Verification items for the finished model (mm, model axes). Face numbers are marked on the shaded views. A direction names the side the tool comes from. Round coordinates to 2 decimals unless told otherwise and drop trailing zeros. Order: outer loops, then holes, each group sorted by start corner. A loop starts at its lowest first (then second) coordinate and runs counter-clockwise, first axis right, second up.
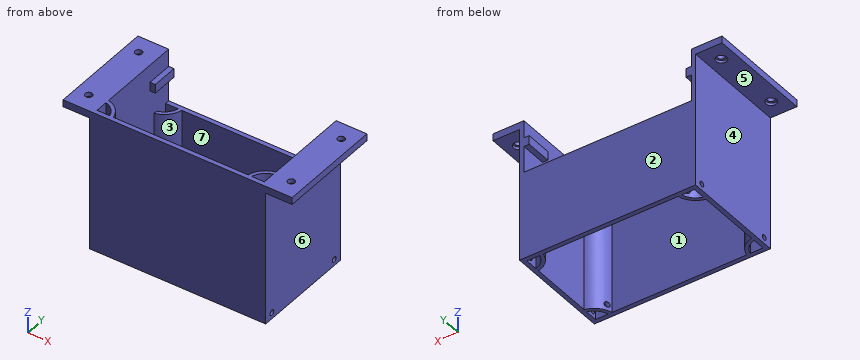
```python
from build123d import *

# Parameters (mm, degrees)
SKETCH1_W                = 100
SKETCH1_H                = 60
SKETCH1_W_2              = 95
SKETCH1_H_2              = 55
BOSS_EXTRUDE1_DEPTH      = 150
SKETCH2_W                = 95
SKETCH2_H                = 30
CUT_EXTRUDE1_DEPTH       = 20
BOSS_EXTRUDE2_DEPTH      = 13
BOSS_EXTRUDE2_DEPTH_BACK = 5
SKETCH3_W                = 106
SKETCH3_H                = 66
SKETCH3_W_2              = 100
SKETCH3_H_2              = 60
SKETCH4_R                = 1.5
CUT_EXTRUDE2_DEPTH       = 120
SKETCH5_R                = 3
CUT_EXTRUDE3_DEPTH       = 1
CUT_EXTRUDE4_START       = -1
SKETCH6_R                = 3
CUT_EXTRUDE4_DEPTH       = 1
SKETCH8_W                = 157.221191822
SKETCH8_H                = 99.5531871
CUT_EXTRUDE6_DEPTH       = 83
SKETCH9_R                = 1.5
CUT_EXTRUDE7_DEPTH       = 120
SKETCH10_W               = 3
SKETCH10_H               = 5
BOSS_EXTRUDE3_DEPTH      = 15
SKETCH11_W               = 15
SKETCH11_H               = 60
SKETCH11_R               = 3
BOSS_EXTRUDE4_DEPTH      = 4
SKETCH11_3_R             = 3
SKETCH11_3_R_2           = 2
BOSS_EXTRUDE5_DEPTH      = 2.5


with BuildPart() as part:
    # Sketch1 → Boss-Extrude1 (new body)
    # profile 1 of 5: a face of its own
    with BuildSketch(Plane.XY):
        with Locations((9.751655629, 0.960264901)):
            Rectangle(SKETCH1_W, SKETCH1_H)
        with Locations((9.751655629, 0.960264901)):
            Rectangle(SKETCH1_W_2, SKETCH1_H_2, mode=Mode.SUBTRACT)
    # profile 2 of 5: a face of its own
    with BuildSketch(Plane.XY):
        with BuildLine():
            Line((-28.511649777, 28.460264901), (-30.565886005, 28.460264901))
            ThreePointArc((-30.565886005, 28.460264901), (-33.177276559, 23.889197089), (-37.748344371, 21.277806535))
            Line((-37.748344371, 21.277806535), (-37.748344371, 19.223570306))
            ThreePointArc((-37.748344371, 19.223570306), (-31.763062997, 22.474983526), (-28.511649777, 28.460264901))
        make_face()
    # profile 3 of 5: a face of its own
    with BuildSketch(Plane.XY):
        with BuildLine():
            Line((50.069197264, 28.460264901), (48.014961035, 28.460264901))
            ThreePointArc((48.014961035, 28.460264901), (51.266374255, 22.474983526), (57.251655629, 19.223570306))
            Line((57.251655629, 19.223570306), (57.251655629, 21.277806535))
            ThreePointArc((57.251655629, 21.277806535), (52.680587817, 23.889197089), (50.069197264, 28.460264901))
        make_face()
    # profile 4 of 5: a face of its own
    with BuildSketch(Plane.XY):
        with BuildLine():
            Line((57.251655629, -19.357276734), (57.251655629, -17.303040505))
            ThreePointArc((57.251655629, -17.303040505), (51.266374255, -20.554453725), (48.014961035, -26.539735099))
            Line((48.014961035, -26.539735099), (50.069197264, -26.539735099))
            ThreePointArc((50.069197264, -26.539735099), (52.680587817, -21.968667287), (57.251655629, -19.357276734))
        make_face()
    # profile 5 of 5: a face of its own
    with BuildSketch(Plane.XY):
        with BuildLine():
            ThreePointArc((-28.511649777, -26.539735099), (-31.763062997, -20.554453725), (-37.748344371, -17.303040505))
            Line((-37.748344371, -17.303040505), (-37.748344371, -19.357276734))
            ThreePointArc((-37.748344371, -19.357276734), (-33.177276559, -21.968667287), (-30.565886005, -26.539735099))
            Line((-30.565886005, -26.539735099), (-28.511649777, -26.539735099))
        make_face()
    extrude(amount=BOSS_EXTRUDE1_DEPTH)

    # Sketch2 → Cut-Extrude1 (cut)
    with BuildSketch(Plane(origin=(0, 30.960264901, 0), x_dir=(1, 0, 0), z_dir=(0, 1, 0))):
        with Locations((9.751655629, -135)):
            Rectangle(SKETCH2_W, SKETCH2_H)
    extrude(amount=-CUT_EXTRUDE1_DEPTH, mode=Mode.SUBTRACT)

    # Sketch3 → Boss-Extrude2 (add, two sides: drawn at the far end of the back side and taken through both)
    with BuildSketch(Plane(origin=(0, 0, 0), x_dir=(-1, 0, 0), z_dir=(0, 0, -1)).offset(-BOSS_EXTRUDE2_DEPTH_BACK)):
        with Locations((-9.751655629, 0.960264901)):
            Rectangle(SKETCH3_W, SKETCH3_H)
        with Locations((-9.751655629, 0.960264901)):
            Rectangle(SKETCH3_W_2, SKETCH3_H_2, mode=Mode.SUBTRACT)
    extrude(amount=BOSS_EXTRUDE2_DEPTH + BOSS_EXTRUDE2_DEPTH_BACK)

    # Sketch4 → Cut-Extrude2 (cut)
    with BuildSketch(Plane.ZY.offset(43.248344371)):
        with Locations((-4, -24.039735099)):
            Circle(SKETCH4_R)
        with Locations((-4, 25.960264901)):
            Circle(SKETCH4_R)
    extrude(amount=-CUT_EXTRUDE2_DEPTH, mode=Mode.SUBTRACT)

    # Sketch5 → Cut-Extrude3 (cut)
    with BuildSketch(Plane(origin=(62.751655629, 0, 0), x_dir=(0, 0, -1), z_dir=(1, 0, 0))):
        with Locations((4, -24.039735099)):
            Circle(SKETCH5_R)
        with Locations((4, 25.960264901)):
            Circle(SKETCH5_R)
    extrude(amount=-CUT_EXTRUDE3_DEPTH, mode=Mode.SUBTRACT)

    # Sketch6 → Cut-Extrude4 (cut)
    with BuildSketch(Plane.ZY.offset(43.248344371).offset(CUT_EXTRUDE4_START)):
        with Locations(Location((-4, 25.960264901, 0), (0, 0, 180))):
            Circle(SKETCH6_R)
        with Locations((-4, -24.087684502)):
            Circle(SKETCH6_R)
    extrude(amount=CUT_EXTRUDE4_DEPTH, mode=Mode.SUBTRACT)

    # Sketch8 → Cut-Extrude6 (cut)
    with BuildSketch(Plane(origin=(0, 0, -13), x_dir=(-1, 0, 0), z_dir=(0, 0, -1))):
        with Locations((-4.996574538, 1.162608777)):
            Rectangle(SKETCH8_W, SKETCH8_H)
    extrude(amount=-CUT_EXTRUDE6_DEPTH, mode=Mode.SUBTRACT)

    # Sketch9 → Cut-Extrude7 (cut)
    with BuildSketch(Plane(origin=(59.751655629, 0, 0), x_dir=(0, 0, -1), z_dir=(1, 0, 0))):
        with Locations(Location((-73.5, -24.039735099, 0), (0, 0, 90))):
            Circle(SKETCH9_R)
        with Locations(Location((-73.5, 25.960264901, 0), (0, 0, 90))):
            Circle(SKETCH9_R)
    extrude(amount=-CUT_EXTRUDE7_DEPTH, mode=Mode.SUBTRACT)

    # Sketch10 → Boss-Extrude3 (add)
    with BuildSketch(Plane(origin=(0, 30.960264901, 0), x_dir=(1, 0, 0), z_dir=(0, 1, 0))):
        with Locations((-36.248344371, -137.5)):
            Rectangle(SKETCH10_W, SKETCH10_H)
        with Locations((55.751655629, -137.5)):
            Rectangle(SKETCH10_W, SKETCH10_H)
    extrude(amount=-BOSS_EXTRUDE3_DEPTH)

    # Sketch11 → Boss-Extrude4 (add)
    # profile 1 of 2: a face of its own
    with BuildSketch(Plane.XY.offset(150)):
        with Locations((-47.748344371, 0.960264901)):
            Rectangle(SKETCH11_W, SKETCH11_H)
        with Locations((-47.748344371, 20.960264901)):
            Circle(SKETCH11_R, mode=Mode.SUBTRACT)
        with Locations((-47.748344371, -19.039735099)):
            Circle(SKETCH11_R, mode=Mode.SUBTRACT)
    # profile 2 of 2: a face of its own
    with BuildSketch(Plane.XY.offset(150)):
        with Locations((67.251655629, 0.960264901)):
            Rectangle(SKETCH11_W, SKETCH11_H)
        with Locations((67.251655629, -19.039735099)):
            Circle(SKETCH11_R, mode=Mode.SUBTRACT)
        with Locations((67.251655629, 20.960264901)):
            Circle(SKETCH11_R, mode=Mode.SUBTRACT)
    extrude(amount=-BOSS_EXTRUDE4_DEPTH)

    # Sketch11_3 → Boss-Extrude5 (add)
    # profile 1 of 4: a face of its own
    with BuildSketch(Plane.XY.offset(150)):
        with Locations((-47.748344371, -19.039735099)):
            Circle(SKETCH11_3_R)
        with Locations((-47.748344371, -19.039735099)):
            Circle(SKETCH11_3_R_2, mode=Mode.SUBTRACT)
    # profile 2 of 4: a face of its own
    with BuildSketch(Plane.XY.offset(150)):
        with Locations((-47.748344371, 20.960264901)):
            Circle(SKETCH11_3_R)
        with Locations((-47.748344371, 20.960264901)):
            Circle(SKETCH11_3_R_2, mode=Mode.SUBTRACT)
    # profile 3 of 4: a face of its own
    with BuildSketch(Plane.XY.offset(150)):
        with Locations((67.251655629, 20.960264901)):
            Circle(SKETCH11_3_R)
        with Locations((67.251655629, 20.960264901)):
            Circle(SKETCH11_3_R_2, mode=Mode.SUBTRACT)
    # profile 4 of 4: a face of its own
    with BuildSketch(Plane.XY.offset(150)):
        with Locations((67.251655629, -19.039735099)):
            Circle(SKETCH11_3_R)
        with Locations((67.251655629, -19.039735099)):
            Circle(SKETCH11_3_R_2, mode=Mode.SUBTRACT)
    extrude(amount=-BOSS_EXTRUDE5_DEPTH)


solid = part.part
```
1) Tool access check on the marked faces 1, 2, 3 and 4. Record the directions out of +Z, -Z, +X, -X, +Y, -Y that give a thin tool (end or side, any length) a straight path to the whole face; none if there is none.
2) Scan lines: probe 1 along X at (y, z) = (6, 114.5); probe 2 along Y at (x, z) = (13, 101); probe 3 along Y at (x, z) = (50, 83.5). Record each from-to range of solid material in increasing order.
3) Sectioned sample at A-A on y = 7. Record the cut outline in (x, z).
4) Go/stop test with flat-tipped pins: pin 1 Ø3 at (x, z) = (50, 136) entering from +Y; pin 2 Ø6.5 at (x, y) = (-46.5, -19.5) entering from -Z; pin 3 Ø2.5 at (y, z) = (24, 137.5) entering from -X; pin 4 Ø2.5 at (x, y) = (-37, 24.5) entering from +Z. Record where each tip stops, or that it passes through.
5) Sectioned sample at B-B on x = -7.5. Record the cut outline in (y, z).
6) Sectioned sample at C-C on z = 107.5. Record the cut outline in (x, y), then the cut area to 3 significant figures.
7) Sectioned sample at D-D on z = 73.5. Count the separate pieces of the cut face and the enclosed holes in it, then the cut area to 3 significant figures.
8) Draft check along X on the marked faces 5, 6 and 7. Enter one of: released by +X, released by -X, zero draft, split by the parting line, or undercut.
Returned:
1. face 1: +Z, -Z
1. face 2: +Z, -Z, +X, -X, +Y
1. face 3: -Z
1. face 4: -Z, -X, +Y, -Y
2. probe 1: x = -40.25 to -37.75, 57.25 to 59.75
2. probe 2: y = -29.04 to -26.54, 28.46 to 30.96
2. probe 3: y = -29.04 to -22.05, 23.97 to 30.96
3. outline: (-55.25, 146) - (-40.25, 146) - (-40.25, 70) - (-37.75, 70) - (-37.75, 150) - (-55.25, 150) - close; (57.25, 70) - (59.75, 70) - (59.75, 146) - (74.75, 146) - (74.75, 150) - (57.25, 150) - close
4. pin 1: stops at y = -20.33
4. pin 2: stops at z = 146
4. pin 3: stops at x = -40.25
4. pin 4: stops at z = 150
5. outline: (-29.04, 70) - (-26.54, 70) - (-26.54, 150) - (-29.04, 150) - close; (28.46, 70) - (30.96, 70) - (30.96, 120) - (28.46, 120) - close
6. outline: (-40.25, -29.04) - (59.75, -29.04) - (59.75, 30.96) - (-40.25, 30.96) - close; hole (-37.75, -26.54) - (-30.57, -26.54) arc R10 ccw to (-37.75, -19.36) - close; hole (-37.75, -17.3) arc R12 cw to (-28.51, -26.54) - (48.01, -26.54) arc R12 cw to (57.25, -17.3) - (57.25, 19.22) arc R12 cw to (48.01, 28.46) - (-28.51, 28.46) arc R12 cw to (-37.75, 19.22) - close; hole (-37.75, 21.28) arc R10 ccw to (-30.57, 28.46) - (-37.75, 28.46) - close; hole (50.07, -26.54) - (57.25, -26.54) - (57.25, -19.36) arc R10 ccw to start; hole (50.07, 28.46) arc R10 ccw to (57.25, 21.28) - (57.25, 28.46) - close
6. area: 873 mm2
7. separate pieces: 4
7. enclosed holes: 0
7. area: 816 mm2
8. face 5: zero draft
8. face 6: released by +X
8. face 7: undercut
